Check sheet for the modelled part. Datum: model origin and axes. Units: mm. Coordinates: 2 decimals unless noted, no trailing zeros. Loops run counter-clockwise (first coordinate to the right, second up) from the corner with the lowest first, then second, coordinate; pieces in that order, holes last. Notation, with made-up numbers: (12.25, -21) -> (69.25, -21) arc R26 cw to (69.25, 6) -> close; hole circle Ø10 at (1, -35.5). An arc over 180 degrees is marked (long way). Use one line per item in the form item = value.
Autodesk Inventor part; units mm, degrees
ref_plane "YZ Plane" through (0, 0, 0) normal (1, 0, 0) x (0, 1, 0)
ref_plane "XZ Plane" through (0, 0, 0) normal (0, 1, 0) x (-1, 0, 0)
ref_plane "XY Plane" through (0, 0, 0) normal (0, 0, 1) x (1, 0, 0)
sketch "Skizze1" plane through (0, 0, 0) normal (0, 0, 1) x (1, 0, 0)
  line L0 (0, 0) -> (15, 0) construction
  line L1 (9, 0) -> (9, -3) construction
  arc A0 (0, 4) -> (-1.2649, -3.7947) centre (0, 0) ccw
  arc A1 (7.7351, -6.7947) -> (10.7889, -6.5777) centre (9, -3) ccw
  arc A2 (16.7889, -3.5777) -> (15, 4) centre (15, 0) ccw
  line L2 (0, 4) -> (15, 4)
  line L3 (16.7889, -3.5777) -> (10.7889, -6.5777)
  line L4 (7.7351, -6.7947) -> (-1.2649, -3.7947)
  dimension "d0" = 4
  dimension "d1" = 15
  dimension "d2" = 3
  dimension "d6" = 9
ref_plane "Arbeitsebene1" through (0, 0, 0) normal (0, 0, -1) x (1, 0, 0)
extrude "Extrusion1" add sketch "Skizze1" along normal blind 3
sketch "Skizze2" plane through (0, 0, 3) normal (0, 0, 1) x (1, 0, 0)
  arc A0 (0, 4) -> (-1.2649, -3.7947) centre (0, 0) ccw
  arc A1 (7.7351, -6.7947) -> (10.7889, -6.5777) centre (9, -3) ccw
  arc A2 (16.7889, -3.5777) -> (15, 4) centre (15, 0) ccw
hole "Bohrung1" at (9, -3, 3) at (15, 0, 3) at (0, 0, 3) direction (0, 0, -1) diameter 3 end through all
sketch "Skizze3" plane through (0, 0, 3) normal (0, 0, 1) x (1, 0, 0)
  circle A0 centre (0, 0) radius 1.5
  arc A1 (0, 4) -> (-1.2649, -3.7947) centre (0, 0) ccw
  circle A2 centre (0, 0) radius 4
extrude "Extrusion2" add sketch "Skizze3" along normal blind 2.6
equation "\"d0\" = bearingWall"
equation "\"d1\" = Hebel_basis_2"
equation "\"d6\" = 0.6 * d1"
equation "\"d4\" = Join_width"
equation "\"d7\" = bearingHole"
equation "\"FingerLaenge_B\" = 25"
equation "\"Hebel_B\" = 25"
equation "\"Finger_width\" = 22"
equation "\"Finger_diameter\" = 8"
equation "\"FingerWall\" = 3"
equation "\"Hebel_basis_2\" = 15"
equation "\"Join_width\" = 3"
equation "\"bearingHole\" = 3"
equation "\"bearingWall\" = 4"
equation "\"support_D\" = 0.25"
properties part number "FingerTip_Mount dual"
(1) Scan lines: line 1 along X through (y, z) = (0, 2.2); line 2 along X through (y, z) = (0, 4); line 3 along Y through (x, z) = (9, 0.8). Record each from-to range of solid material in increasing order.
Established:
line_1 = -4 to -1.5, 1.5 to 13.5, 16.5 to 19
line_2 = -4 to -1.5, 1.5 to 4
line_3 = -7 to -4.5, -1.5 to 4
(2) Mould release check, pull along X, two halves, no side actions. Record for faces 1 (the flat face through (11, -1, 3)), 2 (the flat face through (3.298, -5.316, 1.479)), 3 (the cylindrical face through (10.464, -2.675, 1.479)): +X half, -X half, draft (parallel to the pull), parting line (faces both ways), or undercut.
Established:
face_1 = draft
face_2 = -X half
face_3 = undercut
(3) Go/stop test with flat-tipped pins: P1, Ø2, axis at y = -4.5, z = 5, coming from the +X side; P2, Ø4, axis at x = 15, y = 0, coming from the +Z side; P3, Ø1.5, axis at y = 3, z = 3.5, coming from the +X side. Record where each tip stops, or that it passes through.
Established:
P1 = 1.94
P2 = 3
P3 = 18.17
(4) Section check B-B, the plane z = 2.25. Record the boundary of the cut face in (x, y).
Established:
outline = (-1.26, -3.79) -> (7.74, -6.79) arc R4 ccw to (10.79, -6.58) -> (16.79, -3.58) arc R4 ccw to (15, 4) -> (0, 4) arc R4 ccw to start; hole circle Ø3 at (0, 0); hole circle Ø3 at (9, -3); hole circle Ø3 at (15, 0)
(5) Section check D-D, the plane y = 0.5. Record the boundary of the cut face in (x, z), plus the area to 3 significant figures.
Established:
outline = (-3.97, 0) -> (-1.41, 0) -> (-1.41, 5.6) -> (-3.97, 5.6) -> close; (1.41, 0) -> (13.59, 0) -> (13.59, 3) -> (3.97, 3) -> (3.97, 5.6) -> (1.41, 5.6) -> close; (16.41, 0) -> (18.97, 0) -> (18.97, 3) -> (16.41, 3) -> close
area = 65.1 mm²
(6) Section check C-C, the plane y = -3. Record the boundary of the cut face in (x, z), plus the area to 3 significant figures.
Established:
outline = (-2.65, 0) -> (7.5, 0) -> (7.5, 3) -> (2.65, 3) -> (2.65, 5.6) -> (-2.65, 5.6) -> close; (10.5, 0) -> (17.65, 0) -> (17.65, 3) -> (10.5, 3) -> close
area = 65.6 mm²
(7) Section check A-A, the plane x = 9. Record the boundary of the cut face in (y, z), plus the area to 3 significant figures.
Established:
outline = (-7, 0) -> (-4.5, 0) -> (-4.5, 3) -> (-7, 3) -> close; (-1.5, 0) -> (4, 0) -> (4, 3) -> (-1.5, 3) -> close
area = 24.0 mm²
